CAD build for the part. Positions are in the model's coordinates, mm. Give positions to 0.01 mm unless a question says otherwise; leave off trailing zeros. Write each loop counter-clockwise with the first axis right and the second up, starting at its lowest first coordinate (ties: lowest second). Pieces come first, ordered by that corner, then holes. Notation, with made-up numbers: (26.25, -5.75) - (33.25, -5.75) arc R30 cw to (33.25, 16.25) - close; hole circle Ø5 at (8, 13). An arc over 180 degrees is marked (long way). Answer as a JSON object with one key per item and string values.
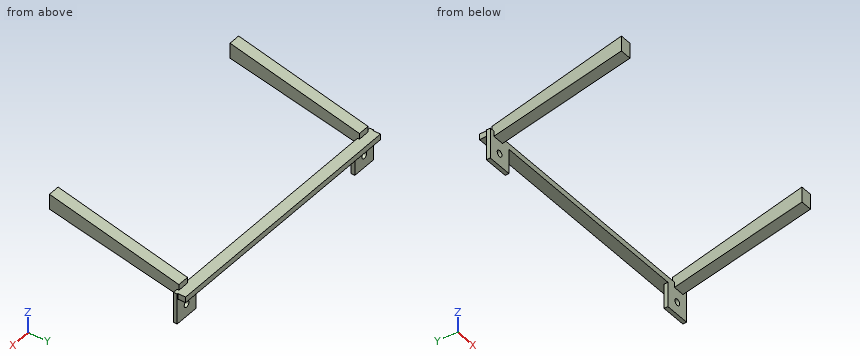
from build123d import *

# Parameters (mm, degrees)
SKETCH_1_W                    = 136
SKETCH_1_H                    = 6
F_3MM_DEPTH                   = 3
EXTRUDE_START                 = -13
SKETCH_2_W                    = 13
SKETCH_2_H                    = 2
EXTRUDE_1_DEPTH               = 16
CUT_EXTRUDE_M3_1_DEPTH        = 100
CUT_EXTRUDE_M3_1_DEPTH_BACK   = 100
SKETCH_3_R                    = 1.65
SKETCH_4_W                    = 13
SKETCH_4_H                    = 2
EXTRUDE_1_2_DEPTH             = 16
CUT_EXTRUDE_M3_1_2_DEPTH      = 100
CUT_EXTRUDE_M3_1_2_DEPTH_BACK = 100
SKETCH_5_R                    = 1.65
F_6MM_1_START                 = -66
F_6MM_1_DEPTH                 = 6
F_6MM_1_START_2               = 60
F_6MM_1_2_DEPTH               = 6


with BuildPart() as part:
    # Sketch 1 → 3mm (new body)
    with BuildSketch(Plane.XY):
        with Locations((0, 81.5)):
            Rectangle(SKETCH_1_W, SKETCH_1_H)
    extrude(amount=F_3MM_DEPTH)

    # Sketch 2 → Extrude 1 (add)
    with BuildSketch(Plane.XY.offset(EXTRUDE_START)):
        with Locations((-62, 79.5)):
            Rectangle(SKETCH_2_W, SKETCH_2_H)
    extrude(amount=EXTRUDE_1_DEPTH)

    # Sketch 3 → Cut-Extrude M3_-1 (cut, two sides: drawn at the far end of the back side and taken through both)
    with BuildSketch(Plane(origin=(0, 0, 0), x_dir=(1, 0, 0), z_dir=(0, 1, 0)).offset(-CUT_EXTRUDE_M3_1_DEPTH_BACK)):
        with Locations(Location((-62, 6.5, 0), (0, 0, 270))):
            Circle(SKETCH_3_R)
    extrude(amount=CUT_EXTRUDE_M3_1_DEPTH + CUT_EXTRUDE_M3_1_DEPTH_BACK, mode=Mode.SUBTRACT)

    # Sketch 4 → Extrude 1 2 (add)
    with BuildSketch(Plane.XY.offset(EXTRUDE_START)):
        with Locations((62, 79.5)):
            Rectangle(SKETCH_4_W, SKETCH_4_H)
    extrude(amount=EXTRUDE_1_2_DEPTH)

    # Sketch 5 → Cut-Extrude M3_1 2 (cut, two sides: drawn at the far end of the back side and taken through both)
    with BuildSketch(Plane(origin=(0, 0, 0), x_dir=(1, 0, 0), z_dir=(0, 1, 0)).offset(-CUT_EXTRUDE_M3_1_2_DEPTH_BACK)):
        with Locations(Location((62, 6.5, 0), (0, 0, 270))):
            Circle(SKETCH_5_R)
    extrude(amount=CUT_EXTRUDE_M3_1_2_DEPTH + CUT_EXTRUDE_M3_1_2_DEPTH_BACK, mode=Mode.SUBTRACT)

    # Sketch 6 → 6mm_-1 (add)
    with BuildSketch(Plane(origin=(0, 0, 0), x_dir=(0, 0, -1), z_dir=(1, 0, 0)).offset(F_6MM_1_START)):
        Polygon((0, 79.5), (-6, 79.5), (-22, 12), (-14, 12), align=None)
    extrude(amount=F_6MM_1_DEPTH)

    # Sketch 7 → 6mm_1 2 (add)
    with BuildSketch(Plane(origin=(0, 0, 0), x_dir=(0, 0, -1), z_dir=(1, 0, 0)).offset(F_6MM_1_START_2)):
        Polygon((0, 79.5), (-6, 79.5), (-22, 12), (-14, 12), align=None)
    extrude(amount=F_6MM_1_2_DEPTH)


solid = part.part
(1) Saw through at B-B, the plane x = 62. Give the cut face in (y, z).
Answer key:
{"outline": "(12, 14) - (78.5, 0.21) - (78.5, -4.85) - (80.5, -4.85) - (80.5, 0) - (84.5, 0) - (84.5, 3) - (79.5, 3) - (79.5, 6) - (12, 22) - close; (78.5, -13) - (80.5, -13) - (80.5, -8.15) - (78.5, -8.15) - close"}
(2) Saw through at C-C, the plane y = 24.5. Give the cut face in (x, z), and give its area (3 significant figures).
Answer key:
{"outline": "(-66, 11.41) - (-60, 11.41) - (-60, 19.04) - (-66, 19.04) - close; (60, 11.41) - (66, 11.41) - (66, 19.04) - (60, 19.04) - close", "area": "91.6 mm²"}
(3) Saw through at A-A, the plane z = -6.5. Give the cut face in (x, y), and give its area (3 significant figures).
Answer key:
{"outline": "(-68.5, 78.5) - (-63.65, 78.5) - (-63.65, 80.5) - (-68.5, 80.5) - close; (-60.35, 78.5) - (-55.5, 78.5) - (-55.5, 80.5) - (-60.35, 80.5) - close; (55.5, 78.5) - (60.35, 78.5) - (60.35, 80.5) - (55.5, 80.5) - close; (63.65, 78.5) - (68.5, 78.5) - (68.5, 80.5) - (63.65, 80.5) - close", "area": "38.8 mm²"}
(4) Probe L1, parallel to X at y = 79.1, z = -6.5; L2, parallel to X at y = 20, z = 14.5; L3, parallel to Z at x = -62, y = 79.6. List the from-to ranges inside material, lowest first. Write a range as [from, to].
Answer key:
{"L1": "x = [-68.5, -63.65], [-60.35, -55.5], [55.5, 60.35], [63.65, 68.5]", "L2": "x = [-66, -60], [60, 66]", "L3": "z = [-13, -8.15], [-4.85, 3]"}
(5) Flat gauge pins, fed straight in: P1, Ø17.5, axis at y = 48, z = 9.5, coming from the -X side; P2, Ø1.8, axis at x = -32.5, y = 82, coming from the +Z side; P3, Ø6.5, axis at x = 24.5, y = 80, coming from the -Z side. Where does each tip first touch, or does it go through?
Answer key:
{"P1": "stops at x = -66", "P2": "stops at z = 3", "P3": "stops at z = 0"}
(6) Saw through at D-D, the plane z = 18.5. Give the cut face in (x, y).
Answer key:
{"outline": "(-66, 12) - (-60, 12) - (-60, 26.77) - (-66, 26.77) - close; (60, 12) - (66, 12) - (66, 26.77) - (60, 26.77) - close"}
